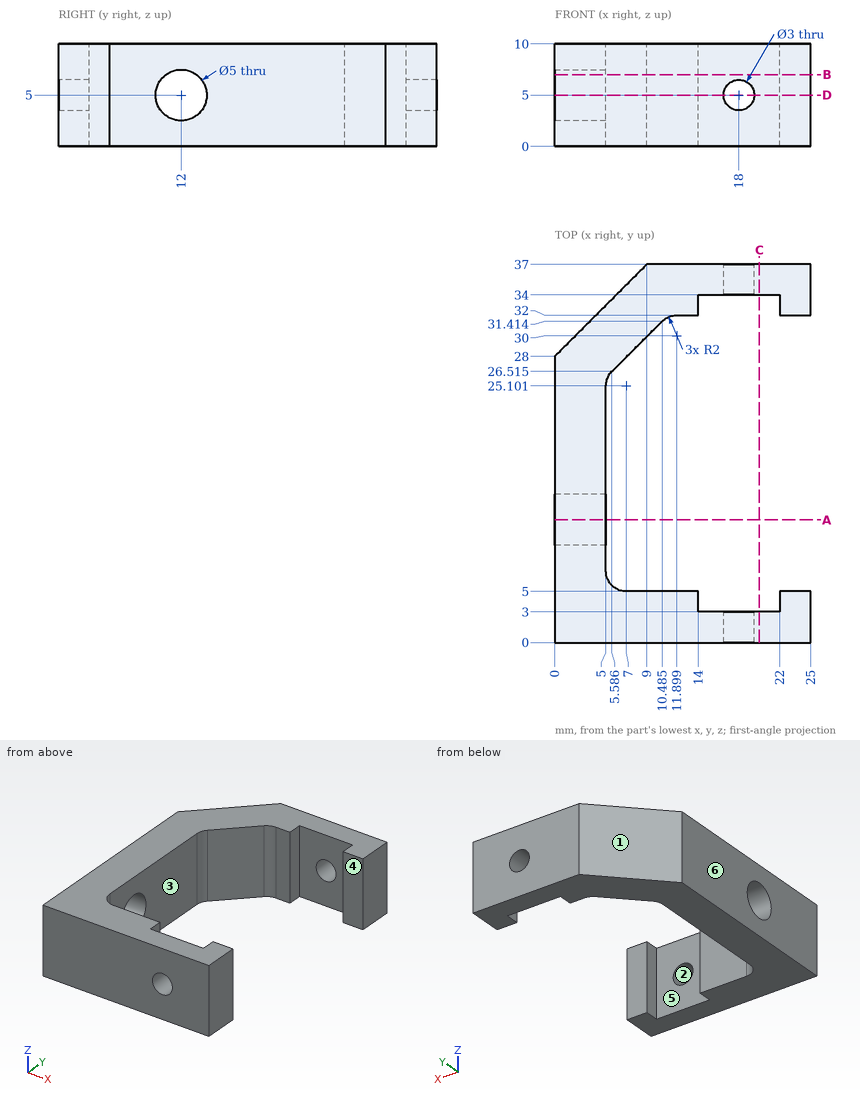
For this review, use the dimensioned drawing (mm, ordinates from the lowest corner) and the shaded views. A direction names the side the tool comes from. Coordinates: 2 decimals unless noted, no trailing zeros. Order: outer loops, then holes, each group sorted by start corner. A loop starts at its lowest first (then second) coordinate and runs counter-clockwise, first axis right, second up. Notation, with made-up numbers: (-8.5, 56) - (22.5, 56) arc R21 ccw to (22.5, 86) - close; hole circle Ø6 at (18, -25). An arc over 180 degrees is marked (long way). Answer as a JSON object with one key per item and string values. Group by question number.
1. For probe 1 along Y at (x, z) = (18.75, 9.25); probe 2 along Z at (x, y) = (4, 10); probe 3 along Y at (x, z) = (23.5, 4.5), list the stretches that pass through material, from the lowest coordinate up.
2. The part is to be moulded in two halves that separate along Y. For the marked faces 1, 2 and 3, say which applies: pulls with the +Y half, pulls with the -Y half, needs draft (parallel to the pull), parting line crosses it, or undercut.
3. We need section B-B on z = 7. State the section outline as (x, y) points (1 decimal), then the cut area to 3 significant figures.
4. For the marked faces 4, 5 and 6, list the 3-axis set-ups (+Z, -Z, +X, -X, +Y, -Y) from which the entire face can be reached by the end or side of a thin tool; tool diameter is ignored.
5. We need section D-D on z = 5. Give the number of separate pieces and of enclosed holes in the cut face, then the cut area to 3 significant figures.
6. We need section A-A on y = 12. State the section outline as (x, z) points.
7. We need section C-C on x = 20. State the section outline as (y, z) points.
8. Clearance check with flat-ended pins moving along their axes: P1, Ø1, axis at y = 33, z = 2.5, coming from the -X side; P2, Ø5, axis at y = 26.5, z = 6.5, coming from the +X side; P3, Ø5, axis at y = 16.5, z = 4.5, coming from the +X side. State where each tip first meets the part, or that it passes through.
Final values:
{
 "1": {"probe 1": "0 to 3, 34 to 37", "probe 2": "0 to 3.5, 6.5 to 10", "probe 3": "0 to 5, 32 to 37"},
 "2": {"face 1": "pulls with the +Y half", "face 2": "needs draft", "face 3": "undercut"},
 "3": {"outline": "(0, 0) - (25, 0) - (25, 5) - (22, 5) - (22, 3) - (14, 3) - (14, 5) - (7, 5) arc R2 cw to (5, 7) - (5, 10.5) - (0, 10.5) - close; (0, 13.5) - (5, 13.5) - (5, 25.1) arc R2 cw to (5.6, 26.5) - (10.5, 31.4) arc R2 cw to (11.9, 32) - (14, 32) - (14, 34) - (22, 34) - (22, 32) - (25, 32) - (25, 37) - (9, 37) - (0, 28) - close", "area": "317 mm²"},
 "4": {"face 4": "+Z, -Z, +X", "face 5": "+Z, -Z", "face 6": "+Z, -Z, -X, +Y, -Y"},
 "5": {"separate pieces": "4", "enclosed holes": "0", "area": "289 mm²"},
 "6": {"outline": "(0, 0) - (5, 0) - (5, 2.5) - (0, 2.5) - close; (0, 7.5) - (5, 7.5) - (5, 10) - (0, 10) - close"},
 "7": {"outline": "(0, 0) - (3, 0) - (3, 10) - (0, 10) - close; (34, 0) - (37, 0) - (37, 10) - (34, 10) - close"},
 "8": {"P1": "x = 4.5", "P2": "x = 8.07", "P3": "x = 5"}
}
